from build123d import *

# Parameters (mm, degrees)
SKETCH2_R           = 1.6
BOSS_EXTRUDE2_DEPTH = 3
FILLET1_R           = 2.5
FILLET2_R           = 0.5


with BuildPart() as part:
    # Sketch2 → Boss-Extrude2 (new body)
    with BuildSketch(Plane.XY):
        with BuildLine():
            Line((9.8, 0.9), (9.8, -5))
            Line((9.8, -5), (17.7, -5))
            Line((17.7, -5), (17.7, 5))
            Line((17.7, 5), (-17.7, 5))
            Line((-17.7, 5), (-17.7, -5))
            Line((-17.7, -5), (-9.8, -5))
            Line((-9.8, -5), (-9.8, 0.9))
            Line((-9.8, 0.9), (-2.878801834, 0.9))
            ThreePointArc((-2.878801834, 0.9), (0, -2.35), (2.878801834, 0.9))
            Line((2.878801834, 0.9), (9.8, 0.9))
        make_face()
        with Locations((0, 0.55)):
            Circle(SKETCH2_R, mode=Mode.SUBTRACT)
    extrude(amount=BOSS_EXTRUDE2_DEPTH)

    # Fillet1
    fillet1_edges = [part.edges().sort_by_distance(p)[0] for p in [
        (-6.339400917, 0.9, 0),
        (6.339400917, 0.9, 0),
    ]]
    fillet(fillet1_edges, radius=FILLET1_R)

    # Fillet2
    fillet2_edges = [part.edges().sort_by_distance(p)[0] for p in [
        (-9.8, -5, 1.5),
        (9.8, -5, 1.5),
    ]]
    fillet(fillet2_edges, radius=FILLET2_R)


solid = part.part
Design review of the part built by this model. Coordinates are the model's own, in mm. Coordinates: 2 decimals unless noted, no trailing zeros. Loops run counter-clockwise (first coordinate to the right, second up) from the corner with the lowest first, then second, coordinate; pieces in that order, holes last. Notation, with made-up numbers: (-24, -18) -> (30, -18) arc R8 cw to (30, -14) -> close; hole circle Ø8 at (-3.5, -31.5). An arc over 180 degrees is marked (long way). Use a Markdown table: item, result. Add a question column.
Item 1: The part is to be moulded in two halves that separate along Y. For faces 1 (the flat face through (-0.2, 2.3, 0)), 2 (the flat face through (14, -5, 1)), 3 (the cylindrical face through (-0.35, -1.01, 1.48)), say which applies: +Y half, -Y half, draft (parallel to the pull), parting line (faces both ways), or undercut.
Item 2: Clearance check with flat-ended pins moving along their axes: P1, Ø1, axis at x = 4, y = -1.5, coming from the -Z side; P2, Ø0.6, axis at x = -6.5, z = 3, coming from the -Y side. State where each tip first meets the part, or that it passes through.
Item 3: We need section A-A, the plane y = 0.55. Write out the cut boundary in (x, z).
Item 4: Wall thickness on L1, parallel to X at y = -2, z = 0.55; L2, parallel to Y at x = 0, z = 2.45; L3, parallel to X at y = -1.75, z = 1.55: over which ranges is each line inside the solid? List them lowest first. Write a range as from..to.
Item 5: We need section D-D, the plane x = -5.5. Write out the cut boundary in (y, z).
Item 6: We need section C-C, the plane z = 1.05. Write out the cut boundary in (x, y).
Item 7: We need section B-B, the plane x = 0. Write out the cut boundary in (y, z), and give its area (4 significant figures).
Numbers:
| question | item | result |
|---|---|---|
| 1 | face 1 | draft |
| 1 | face 2 | -Y half |
| 1 | face 3 | undercut |
| 2 | P1 | passes through |
| 2 | P2 | stops at y = 0.9 |
| 3 | outline | (-17.7, 0) -> (-9.8, 0) -> (-9.8, 3) -> (-17.7, 3) -> close; (-2.9, 0) -> (-1.6, 0) -> (-1.6, 3) -> (-2.9, 3) -> close; (1.6, 0) -> (2.9, 0) -> (2.9, 3) -> (1.6, 3) -> close; (9.8, 0) -> (17.7, 0) -> (17.7, 3) -> (9.8, 3) -> close |
| 4 | L1 | x = -17.7..-9.8, -1.38..1.38, 9.8..17.7 |
| 4 | L2 | y = -2.35..-1.05, 2.15..5 |
| 4 | L3 | x = -17.7..-9.8, -1.77..1.77, 9.8..17.7 |
| 5 | outline | (0.9, 2.5) arc R2.5 ccw to (3.4, 0) -> (5, 0) -> (5, 3) -> (0.9, 3) -> close |
| 6 | outline | (-17.7, -5) -> (-10.3, -5) arc R0.5 ccw to (-9.8, -4.5) -> (-9.8, 1.36) -> (-2.78, 1.36) arc R2.9 ccw (long way) to (2.78, 1.36) -> (9.8, 1.36) -> (9.8, -4.5) arc R0.5 ccw to (10.3, -5) -> (17.7, -5) -> (17.7, 5) -> (-17.7, 5) -> close; hole circle Ø3.2 at (0, 0.55) |
| 7 | outline | (-2.35, 0) -> (-1.05, 0) -> (-1.05, 3) -> (-2.35, 3) -> close; (2.15, 0) -> (5, 0) -> (5, 3) -> (2.15, 3) -> close |
| 7 | area | 12.45 mm^2 |
